```python
from build123d import *

# Parameters (mm, degrees)
SKETCH1_W           = 300
SKETCH1_H           = 150
BOSS_EXTRUDE1_DEPTH = 19.05
SKETCH1_3_W         = 19.05
SKETCH1_3_H         = 150
CUT_EXTRUDE1_DEPTH  = 6
SKETCH4_R           = 2
CUT_EXTRUDE3_DEPTH  = 14.05


with BuildPart() as part:
    # Sketch1 → Boss-Extrude1 (new body)
    with BuildSketch(Plane.XY):
        with Locations((150, 75)):
            Rectangle(SKETCH1_W, SKETCH1_H)
    extrude(amount=BOSS_EXTRUDE1_DEPTH)

    # Sketch1_3 → Cut-Extrude1 (cut)
    with BuildSketch(Plane.XY):
        with Locations((181.496, 75)):
            Rectangle(SKETCH1_3_W, SKETCH1_3_H)
        with Locations((118.504, 75)):
            Rectangle(SKETCH1_3_W, SKETCH1_3_H)
    extrude(amount=CUT_EXTRUDE1_DEPTH, mode=Mode.SUBTRACT)

    # Sketch4 → Cut-Extrude3 (cut, through all)
    with BuildSketch(Plane(origin=(0, 0, 6), x_dir=(-1, 0, 0), z_dir=(0, 0, -1))):
        with Locations((-118.504, 30)):
            Circle(SKETCH4_R)
        with Locations((-181.496, 30)):
            Circle(SKETCH4_R)
        with Locations((-181.496, 60)):
            Circle(SKETCH4_R)
        with Locations((-181.496, 90)):
            Circle(SKETCH4_R)
        with Locations((-181.496, 120)):
            Circle(SKETCH4_R)
        with Locations((-118.504, 60)):
            Circle(SKETCH4_R)
        with Locations((-118.504, 90)):
            Circle(SKETCH4_R)
        with Locations((-118.504, 120)):
            Circle(SKETCH4_R)
    extrude(amount=-CUT_EXTRUDE3_DEPTH, mode=Mode.SUBTRACT)


solid = part.part
```
The model under review builds one solid part; all positions refer to its coordinate system, in mm. A direction names the side the tool comes from. Give positions to 0.01 mm unless a question says otherwise; leave off trailing zeros. Order: outer loops, then holes, each group sorted by start corner. A loop starts at its lowest first (then second) coordinate and runs counter-clockwise, first axis right, second up. Notation, with made-up numbers: (66.5, 60.25) - (90.5, 60.25) arc R7 ccw to (90.5, 64.25) - close; hole circle Ø9 at (-8, 89.25). An arc over 180 degrees is marked (long way). Use CSV: the item, a comma, the result in double quotes. Start each with the question number.
Q1. The part is to be moulded in two halves that separate along X. For faces 1 (the flat face through (181, 76, 6)), 2 (the flat face through (0, 74, 9)), 3 (the flat face through (148, 150, 9)), 4 (the flat face through (108.979, 74, 3)), say which applies: +X half, -X half, draft (parallel to the pull), parting line (faces both ways), or undercut.
Q2. We need section A-A, the plane y = 19. Write out the cut boundary in (x, z).
Q3. We need section B-B, the plane x = 125. Write out the cut boundary in (y, z).
Q4. Clearance check with a flat-ended pin moving along its axis: pin 1 Ø6.5 at (x, y) = (181.496, 30) entering from -Z. State where the tip first meets the part, or that it passes through.
Q5. To check wall thickness, follow line 1 along X through (y, z) = (70.5, 3.25); line 2 along X through (y, z) = (60.5, 7); line 3 along Z through (x, y) = (121, 6.5). State the ranges of each line that lie inside material, in increasing order. Write a range as [from, to].
Q6. Tool access review of faces 5 (the flat face through (300, 74, 9)), 6 (the flat face through (171.971, 74, 3)): name each direction out of +Z, -Z, +X, -X, +Y, -Y from which nothing blocks a thin tool from reaching the whole face with its end or side.
Outcome:
1,face 1,"undercut"
1,face 2,"-X half"
1,face 3,"draft"
1,face 4,"undercut"
2,outline,"(0, 0) - (108.98, 0) - (108.98, 6) - (128.03, 6) - (128.03, 0) - (171.97, 0) - (171.97, 6) - (191.02, 6) - (191.02, 0) - (300, 0) - (300, 19.05) - (0, 19.05) - close"
3,outline,"(0, 6) - (150, 6) - (150, 19.05) - (0, 19.05) - close"
4,pin 1,"stops at z = 6"
5,line 1,"x = [0, 108.98], [128.03, 171.97], [191.02, 300]"
5,line 2,"x = [0, 116.57], [120.44, 179.56], [183.43, 300]"
5,line 3,"z = [6, 19.05]"
6,face 5,"+Z, -Z, +X, +Y, -Y"
6,face 6,"-Z, +Y, -Y"
